Design review of the part shown in the three views and the two pictorial views. Dimensions are in mm from the part's minimum x, y and z. Coordinates: 2 decimals unless noted, no trailing zeros. Write each loop counter-clockwise with the first axis right and the second up, starting at its lowest first coordinate (ties: lowest second). Pieces come first, ordered by that corner, then holes. Notation, with made-up numbers: (78, 82) -> (137, 82) arc R23 cw to (137, 93) -> close; hole circle Ø8 at (3, 15.25). An arc over 180 degrees is marked (long way). Write each question's results on one line, items separated by ' | '.
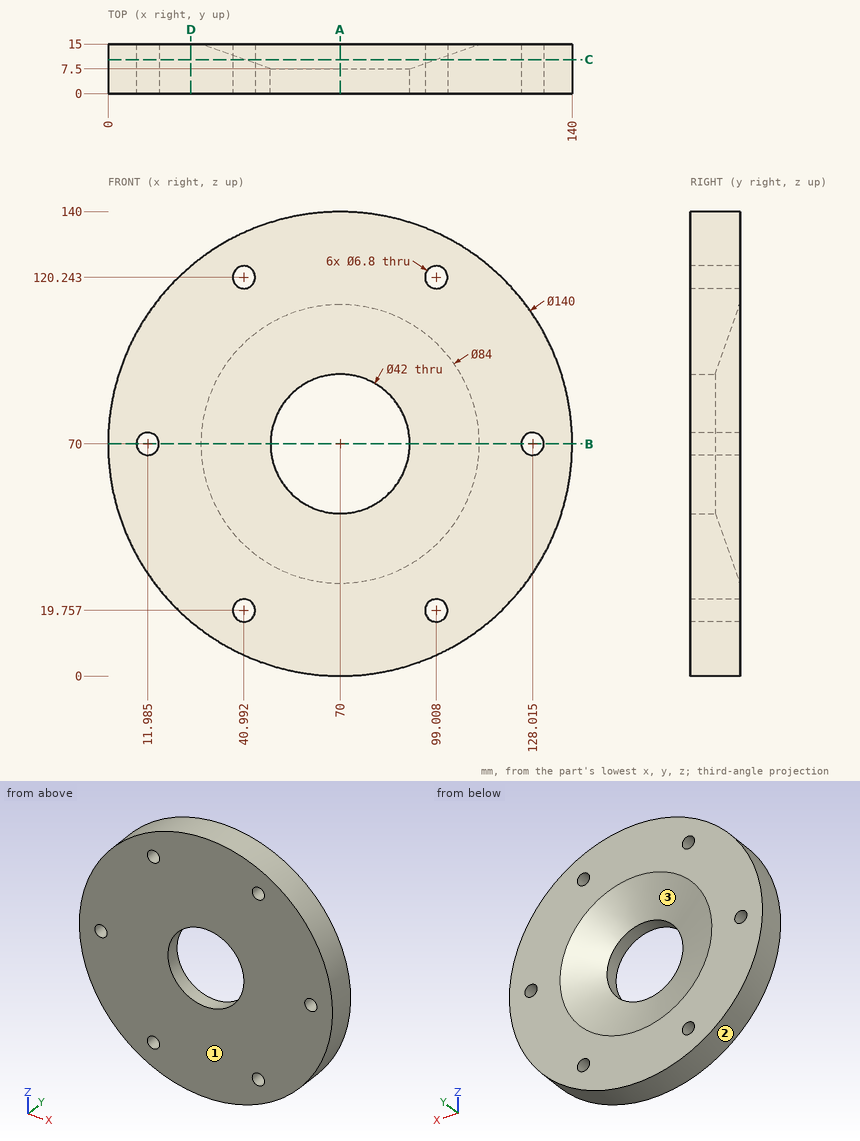
Q1. Draft analysis for pull direction Z (two halves, no side actions). For the marked faces 1, 2 and 3, state which applies: pulls with the +Z half, pulls with the -Z half, needs draft (parallel to the pull), parting line crosses it, or undercut.
Solution:
face 1: needs draft | face 2: parting line crosses it | face 3: undercut
Q2. For line 1 (X direction, y = 7, z = 70) (1 decimal); line 2 (X direction, y = 13.5, z = 20) (1 decimal); line 3 (Z direction, x = 81, y = 6.75), list the stretches that pass through material, from the lowest coordinate up. Write a range as from..to.
Solution:
line 1: 0..8.6, 15.4..49, 91..124.6, 131.4..140 | line 2: 21..37.6, 44.4..95.6, 102.4..119 | line 3: 0.87..52.11, 87.89..139.13
Q3. Add section D-D (x = 25). Write out the cut boundary in (y, z).
Solution:
outline: (0, 16.38) -> (15, 16.38) -> (15, 123.62) -> (0, 123.62) -> close
Q4. Clearance check with flat-ended pins moving along their axes: P1, Ø2, axis at x = 105, y = 2, coming from the -Z side; P2, Ø8, axis at x = 86.5, y = 4.5, coming from the -Z side (1 decimal); P3, Ø3, axis at x = 51.5, y = 4.5, coming from the -Z side (1 decimal). State where each tip first meets the part, or that it passes through.
Solution:
P1: z = 8.81 | P2: z = 1.1 | P3: z = 2.1
Q5. Add section A-A (x = 70). Write out the cut boundary in (y, z).
Solution:
outline: (0, 0) -> (15, 0) -> (15, 28) -> (7.5, 49) -> (0, 49) -> close; (0, 91) -> (7.5, 91) -> (15, 112) -> (15, 140) -> (0, 140) -> close
Q6. Add section C-C (y = 10.25). Write out the cut boundary in (x, z) (1 decimal).
Solution:
outline: circle Ø140 at (70, 70); hole circle Ø6.8 at (12, 70); hole circle Ø6.8 at (41, 19.8); hole circle Ø6.8 at (41, 120.2); hole circle Ø57.4 at (70, 70); hole circle Ø6.8 at (99, 19.8); hole circle Ø6.8 at (99, 120.2); hole circle Ø6.8 at (128, 70)
Q7. Add section B-B (z = 70). Write out the cut boundary in (x, y) (1 decimal).
Solution:
outline: (0, 0) -> (8.6, 0) -> (8.6, 15) -> (0, 15) -> close; (15.4, 0) -> (49, 0) -> (49, 7.5) -> (28, 15) -> (15.4, 15) -> close; (91, 0) -> (124.6, 0) -> (124.6, 15) -> (112, 15) -> (91, 7.5) -> close; (131.4, 0) -> (140, 0) -> (140, 15) -> (131.4, 15) -> close
